from build123d import *

# Parameters (mm, degrees)
F1_DEPTH  = 2.667
F3_D      = 6.0198
F4_D      = 4.7879
F5_D      = 4.0386
F6_W      = 32.8803089343
F6_H      = 42.4424372282
F7_DEPTH  = 0.0127
F8_W      = 27.7899198272
F8_H      = 25.566725319
F9_DEPTH  = 0.0127
F10_R     = 1.016
F11_R     = 0.635
F12_SIZE2 = 1.778
F12_SIZE  = 1.778


with BuildPart() as f1:
    # F0 (on Front) → F1 (new body)
    with BuildSketch(Plane.XZ):
        with BuildLine():
            Line((60.0202, 0), (0, 0))
            Line((0, 0), (0, -12.7))
            Line((0, -12.7), (60.0202, -12.7))
            ThreePointArc((60.0202, -12.7), (64.5103280605, -10.8401280605), (66.3702, -6.35))
            ThreePointArc((66.3702, -6.35), (64.5103280605, -1.8598719395), (60.0202, 0))
        make_face()
    extrude(amount=-F1_DEPTH)

    # F3 (through all)
    with Locations(Plane.XZ):
        with Locations((60.0202, -6.35)):
            Hole(F3_D / 2)

    # F4 (through all)
    with Locations(Plane.XZ):
        with Locations((40.64, -6.35)):
            Hole(F4_D / 2)

    # F5 (through all)
    with Locations(Plane.XZ):
        with Locations((15.24, -6.35)):
            Hole(F5_D / 2)

    # F6 (on face) → F7 (cut)
    with BuildSketch(Plane.XZ):
        with Locations((67.2401544672, -9.9617778324)):
            Rectangle(F6_W, F6_H)
    extrude(amount=-F7_DEPTH, mode=Mode.SUBTRACT)

    # F8 (on face) → F9 (cut)
    with BuildSketch(Plane(origin=(0, 2.667, 0), x_dir=(-1, 0, 0), z_dir=(0, 1, 0))):
        with Locations((-64.6949599136, -4.1028452106)):
            Rectangle(F8_W, F8_H)
    extrude(amount=-F9_DEPTH, mode=Mode.SUBTRACT)

    # F10
    f10_edges = [f1.edges().sort_by_distance(p)[0] for p in [
        (55.4101, 0.0127, -12.7),
    ]]
    fillet(f10_edges, radius=F10_R)

    # F11
    f11_edges = [f1.edges().sort_by_distance(p)[0] for p in [
        (55.4101, 2.6543, 0),
    ]]
    fillet(f11_edges, radius=F11_R)

    # F12
    f12_edges = [f1.edges().sort_by_distance(p)[0] for p in [
        (0, 2.667, -6.35),
    ]]
    chamfer(f12_edges, length=F12_SIZE, length2=F12_SIZE2)


solid = f1.part
Verification items for the finished model (mm, model axes). A direction names the side the tool comes from. Round coordinates to 2 decimals unless told otherwise and drop trailing zeros. Loops run counter-clockwise (first coordinate to the right, second up) from the corner with the lowest first, then second, coordinate; pieces in that order, holes last. Notation, with made-up numbers: (85, 47) - (97, 47) arc R14 cw to (97, 59) - close; hole circle Ø9 at (34.5, 11). An arc over 180 degrees is marked (long way). Use one line per item in the form item = value.
1. Access from +Z, -Z, +X, -X, +Y, -Y to the whole of each face (thin tool, end or side, straight path). Record for faces 5 (the cylindrical face through (55.47, 0.3, -0.31)), 6 (the flat face through (50.8, 0.17, -12.49)), 7 (the flat face through (30, 1, -12.7)).
A:
face_5 = +Z, +X, -Y
face_6 = +X, -Y
face_7 = -Z, +X, -X, +Y, -Y
2. Scan lines: probe 1 along X at (y, z) = (2.25, -6.25); probe 2 along Z at (x, y) = (40.64, 1.65); probe 3 along X at (y, z) = (0.5, -7.25). Record each from-to range of solid material in increasing order.
A:
probe_1 = 1.36 to 13.22, 17.26 to 38.25, 43.03 to 57.01, 63.03 to 66.33
probe_2 = -12.7 to -8.74, -3.96 to 0
probe_3 = 0 to 13.43, 17.05 to 38.42, 42.86 to 57.15, 62.89 to 66.16
3. Section check C-C on x = 15.24. Record the cut outline in (y, z).
A:
outline = (0, -12.7) - (2.67, -12.7) - (2.67, -8.37) - (0, -8.37) - close; (0, -4.33) - (2.67, -4.33) - (2.67, 0) - (0, 0) - close
4. Section check B-B on z = -5.5. Give the number of separate pieces and of enclosed holes in the cut face, and give its area (3 significant figures).
A:
separate_pieces = 4
enclosed_holes = 0
area = 138 mm²
5. Gauge pin test, flat ends, axial feed: pin 1 Ø3 at (x, z) = (15.24, -6.35) entering from -Y; pin 2 Ø3.5 at (x, z) = (58.5, -6) entering from +Y; pin 3 Ø1.5 at (y, z) = (1.5, -11.5) entering from +X; pin 4 Ø0.5 at (y, z) = (0.5, -3.5) entering from +X. Record the tip position at first contact, or that the pin passes through.
A:
pin_1 = through
pin_2 = 2.65
pin_3 = 64.6
pin_4 = 65.71
6. Section check A-A on x = 40.64. Record the cut outline in (y, z).
A:
outline = (0, -12.7) - (2.67, -12.7) - (2.67, -8.74) - (0, -8.74) - close; (0, -3.96) - (2.67, -3.96) - (2.67, 0) - (0, 0) - close
7. Draft check along X on faces 1 (the cylindrical face through (57.15, 1.35, -5.45)), 2 (the flat face through (0.9, 1.79, -6.26)), 3 (the cylindrical face through (55.35, 0.3, -12.39)), 4 (the cylindrical face through (43.03, 1.35, -6.24)). Enter one of: pulls with the +X half, pulls with the -X half, needs draft (parallel to the pull), parting line crosses it, or undercut.
A:
face_1 = undercut
face_2 = pulls with the -X half
face_3 = needs draft
face_4 = undercut
